from build123d import *

# Parameters (mm, degrees)
MODEL_R             = 2.100000001
BOSS_EXTRUDE1_DEPTH = 431.1


with BuildPart() as part:
    # Model → Boss-Extrude1 (new body)
    with BuildSketch(Plane.XY):
        with BuildLine():
            Line((28.771485975, 48.105572105), (30.646485975, 49.980572105))
            ThreePointArc((30.646485975, 49.980572105), (30.808697649, 50.08895848), (31.000039365, 50.127018713))
            Line((31.000039365, 50.127018713), (31.592932584, 50.127018713))
            Line((31.592932584, 50.127018713), (31.592932584, 47.752018713))
            Line((31.592932584, 47.752018713), (38.292932585, 47.752018713))
            ThreePointArc((38.292932585, 47.752018713), (38.505064619, 47.664150748), (38.592932584, 47.452018714))
            Line((38.592932584, 47.452018714), (38.592932584, 45.752018713))
            Line((38.592932584, 45.752018713), (35.592932585, 45.752018713))
            Line((35.592932585, 45.752018713), (35.592932585, 44.812678885))
            Line((35.592932585, 44.812678885), (38.653592756, 41.752018713))
            Line((38.653592756, 41.752018713), (41.292932583, 41.752018713))
            Line((41.292932583, 41.752018713), (41.592932584, 41.452018713))
            Line((41.592932584, 41.452018713), (41.892932586, 41.752018714))
            Line((41.892932586, 41.752018714), (44.532272412, 41.752018714))
            Line((44.532272412, 41.752018714), (47.592932584, 44.812678886))
            Line((47.592932584, 44.812678886), (47.592932584, 45.752018714))
            Line((47.592932584, 45.752018714), (44.592932584, 45.752018714))
            Line((44.592932584, 45.752018714), (44.592932584, 47.452018715))
            ThreePointArc((44.592932584, 47.452018715), (44.68080055, 47.664150749), (44.892932584, 47.752018715))
            Line((44.892932584, 47.752018715), (61.292932583, 47.752018715))
            Line((61.292932583, 47.752018715), (61.592932582, 47.452018715))
            Line((61.592932582, 47.452018715), (61.892932583, 47.752018716))
            Line((61.892932583, 47.752018716), (71.592932583, 47.752018716))
            Line((71.592932583, 47.752018716), (71.592932583, 50.127018711))
            Line((71.592932583, 50.127018711), (72.185825802, 50.127018711))
            ThreePointArc((72.185825802, 50.127018711), (72.377167518, 50.088958477), (72.539379192, 49.980572102))
            Line((72.539379192, 49.980572102), (74.414379192, 48.105572102))
            ThreePointArc((74.414379192, 48.105572102), (74.560825801, 47.752018712), (74.414379192, 47.398465322))
            Line((74.414379192, 47.398465322), (72.539379192, 45.523465322))
            ThreePointArc((72.539379192, 45.523465322), (72.377167518, 45.415078947), (72.185825802, 45.377018714))
            Line((72.185825802, 45.377018714), (72.092932582, 45.377018714))
            ThreePointArc((72.092932582, 45.377018714), (71.739379192, 45.230572103), (71.592932583, 44.877018713))
            Line((71.592932583, 44.877018713), (71.592932583, 41.052018712))
            ThreePointArc((71.592932583, 41.052018712), (71.505064617, 40.839886678), (71.292932581, 40.752018713))
            Line((71.292932581, 40.752018713), (69.592932583, 40.752018713))
            Line((69.592932583, 40.752018713), (69.592932583, 43.752018712))
            Line((69.592932583, 43.752018712), (68.653592755, 43.752018712))
            Line((68.653592755, 43.752018712), (65.592932583, 40.691358541))
            Line((65.592932583, 40.691358541), (65.592932583, 38.052018712))
            Line((65.592932583, 38.052018712), (65.292932584, 37.752018712))
            Line((65.292932584, 37.752018712), (65.592932583, 37.452018713))
            Line((65.592932583, 37.452018713), (65.592932583, 34.812678884))
            Line((65.592932583, 34.812678884), (68.653592755, 31.752018712))
            Line((68.653592755, 31.752018712), (69.592932583, 31.752018712))
            Line((69.592932583, 31.752018712), (69.592932583, 34.752018711))
            Line((69.592932583, 34.752018711), (71.292932581, 34.752018711))
            ThreePointArc((71.292932581, 34.752018711), (71.505064617, 34.664150747), (71.592932583, 34.452018712))
            Line((71.592932583, 34.452018712), (71.592932583, 28.75201871))
            ThreePointArc((71.592932583, 28.75201871), (71.300039364, 28.044911929), (70.592932582, 27.752018711))
            Line((70.592932582, 27.752018711), (64.892932582, 27.752018711))
            ThreePointArc((64.892932582, 27.752018711), (64.680800548, 27.839886676), (64.592932583, 28.05201871))
            Line((64.592932583, 28.05201871), (64.592932583, 29.752018711))
            Line((64.592932583, 29.752018711), (67.592932582, 29.752018711))
            Line((67.592932582, 29.752018711), (67.592932582, 30.69135854))
            Line((67.592932582, 30.69135854), (64.532272411, 33.752018711))
            Line((64.532272411, 33.752018711), (61.892932584, 33.752018711))
            Line((61.892932584, 33.752018711), (61.592932582, 34.052018713))
            Line((61.592932582, 34.052018713), (61.292932582, 33.752018712))
            Line((61.292932582, 33.752018712), (58.653592755, 33.752018712))
            Line((58.653592755, 33.752018712), (55.592932583, 30.691358541))
            Line((55.592932583, 30.691358541), (55.592932583, 29.752018713))
            Line((55.592932583, 29.752018713), (58.592932583, 29.752018713))
            Line((58.592932583, 29.752018713), (58.592932583, 28.052018712))
            ThreePointArc((58.592932583, 28.052018712), (58.505064617, 27.839886678), (58.292932583, 27.752018712))
            Line((58.292932583, 27.752018712), (44.892932584, 27.752018712))
            ThreePointArc((44.892932584, 27.752018712), (44.68080055, 27.839886678), (44.592932584, 28.052018712))
            Line((44.592932584, 28.052018712), (44.592932584, 29.752018713))
            Line((44.592932584, 29.752018713), (47.592932584, 29.752018713))
            Line((47.592932584, 29.752018713), (47.592932584, 30.691358541))
            Line((47.592932584, 30.691358541), (44.532272412, 33.752018712))
            Line((44.532272412, 33.752018712), (41.892932586, 33.752018712))
            Line((41.892932586, 33.752018712), (41.592932584, 34.052018714))
            Line((41.592932584, 34.052018714), (41.292932583, 33.752018714))
            Line((41.292932583, 33.752018714), (38.653592756, 33.752018714))
            Line((38.653592756, 33.752018714), (35.592932585, 30.691358542))
            Line((35.592932585, 30.691358542), (35.592932585, 29.752018714))
            Line((35.592932585, 29.752018714), (38.592932584, 29.752018714))
            Line((38.592932584, 29.752018714), (38.592932584, 28.052018713))
            ThreePointArc((38.592932584, 28.052018713), (38.505064619, 27.839886679), (38.292932585, 27.752018714))
            Line((38.292932585, 27.752018714), (32.592932585, 27.752018714))
            ThreePointArc((32.592932585, 27.752018714), (31.885825803, 28.044911931), (31.592932584, 28.752018713))
            Line((31.592932584, 28.752018713), (31.592932584, 34.452018715))
            ThreePointArc((31.592932584, 34.452018715), (31.68080055, 34.664150748), (31.892932583, 34.752018714))
            Line((31.892932583, 34.752018714), (33.592932584, 34.752018714))
            Line((33.592932584, 34.752018714), (33.592932584, 31.752018715))
            Line((33.592932584, 31.752018715), (34.532272412, 31.752018715))
            Line((34.532272412, 31.752018715), (37.592932584, 34.812678886))
            Line((37.592932584, 34.812678886), (37.592932584, 37.452018715))
            Line((37.592932584, 37.452018715), (37.892932583, 37.752018715))
            Line((37.892932583, 37.752018715), (37.592932584, 38.052018714))
            Line((37.592932584, 38.052018714), (37.592932584, 40.691358543))
            Line((37.592932584, 40.691358543), (34.532272412, 43.752018715))
            Line((34.532272412, 43.752018715), (33.592932584, 43.752018715))
            Line((33.592932584, 43.752018715), (33.592932584, 40.752018716))
            Line((33.592932584, 40.752018716), (31.892932586, 40.752018716))
            ThreePointArc((31.892932586, 40.752018716), (31.68080055, 40.83988668), (31.592932584, 41.052018715))
            Line((31.592932584, 41.052018715), (31.592932584, 44.877018715))
            ThreePointArc((31.592932584, 44.877018715), (31.446485975, 45.230572106), (31.092932585, 45.377018716))
            Line((31.092932585, 45.377018716), (31.000039365, 45.377018716))
            ThreePointArc((31.000039365, 45.377018716), (30.808697649, 45.41507895), (30.646485975, 45.523465324))
            Line((30.646485975, 45.523465324), (28.771485975, 47.398465325))
            ThreePointArc((28.771485975, 47.398465325), (28.625039366, 47.752018715), (28.771485975, 48.105572105))
        make_face()
        with Locations((61.592932582, 37.752018715)):
            Circle(MODEL_R, mode=Mode.SUBTRACT)
        with Locations((41.592932582, 37.752018715)):
            Circle(MODEL_R, mode=Mode.SUBTRACT)
        with BuildLine():
            Line((54.092932584, 29.752018715), (49.092932584, 29.752018715))
            Line((49.092932584, 29.752018715), (49.092932584, 31.312678886))
            Line((49.092932584, 31.312678886), (45.592932583, 34.812678886))
            Line((45.592932583, 34.812678886), (45.592932583, 40.691358543))
            Line((45.592932583, 40.691358543), (49.092932584, 44.191358544))
            Line((49.092932584, 44.191358544), (49.092932584, 45.752018714))
            Line((49.092932584, 45.752018714), (67.592932582, 45.752018714))
            Line((67.592932582, 45.752018714), (67.592932582, 44.812678887))
            Line((67.592932582, 44.812678887), (64.532272411, 41.752018716))
            Line((64.532272411, 41.752018716), (61.402932584, 41.752018716))
            ThreePointArc((61.402932584, 41.752018716), (58.708855747, 40.636095552), (57.592932584, 37.942018716))
            Line((57.592932584, 37.942018716), (57.592932584, 34.812678886))
            Line((57.592932584, 34.812678886), (54.092932584, 31.312678886))
            Line((54.092932584, 31.312678886), (54.092932584, 29.752018715))
        make_face(mode=Mode.SUBTRACT)
    extrude(amount=-BOSS_EXTRUDE1_DEPTH)


solid = part.part
Could you check a few things on this model? Use its own coordinates, in mm. A direction names the side the tool comes from. Round coordinates to 2 decimals unless told otherwise and drop trailing zeros.
Q1. I'm going to push flat-ended pins straight in: P1, Ø5, axis at y = 33.5, z = -344.5, coming from the +X side; P2, Ø8, axis at x = 51.5, z = -270, coming from the +Y side; P3, Ø0.9, axis at y = 47, z = -152.5, coming from the -X side. Where does each tip first touch, or does it pass through?
Geometry says:
P1: stops at x = 71.59
P2: stops at y = 47.75
P3: stops at x = 28.73
Q2. Imagine slicing it at A-A, the plane z = -219. State how many separate pieces and enclosed holes the cut face has, then the cut area to 3 significant figures.
Geometry says:
separate pieces: 1
enclosed holes: 3
area: 341 mm2
Q3. Which directions (+Z, -Z, +X, -X, +Y, -Y) give clear straight access to the entire face, cutting with the end or side of a thin tool? Please do faces 1 (the face through (48, 44, 0)), 2 (the face through (58, 45.752, -213)), 3 (the face through (35, 47.752, -213)).
Geometry says:
face 1: +Z, +X, -X, +Y, -Y
face 2: +Z, -Z
face 3: +Z, -Z, +Y
Q4. Thinking about a two-plate mould opening in X: for faces 4 (the face through (53, 47.752, -213)), 5 (the face through (48, 44, -431.1)), which applies, released by +X, released by -X, zero draft, split by the parting line, or undercut?
Geometry says:
face 4: undercut
face 5: zero draft
Q5. Please list where these lines run through material, in increasing order: probe 1 along X at (y, z) = (30, -142); probe 2 along X at (y, z) = (29.25, -99.5); probe 3 along Y at (x, z) = (38.5, -132.5).
Geometry says:
probe 1: x = 31.59 to 35.59, 47.59 to 49.09, 54.09 to 55.59, 67.59 to 71.59
probe 2: x = 31.59 to 38.59, 44.59 to 58.59, 64.59 to 71.59
probe 3: y = 27.83 to 29.75, 33.6 to 41.91, 45.75 to 47.67
